The listing builds one solid part. Answer for the finished solid, in the listing's coordinates (mm). A direction names the side the tool comes from. Coordinates: 2 decimals unless noted, no trailing zeros. Write each loop counter-clockwise with the first axis right and the second up, starting at its lowest first coordinate (ties: lowest second). Pieces come first, ordered by that corner, then holes.
Autodesk Inventor part; units mm, degrees
ref_plane "YZ Plane" through (0, 0, 0) normal (1, 0, 0) x (0, 1, 0)
ref_plane "XZ Plane" through (0, 0, 0) normal (0, 1, 0) x (-1, 0, 0)
ref_plane "XY Plane" through (0, 0, 0) normal (0, 0, 1) x (1, 0, 0)
sketch "Sketch1" plane through (0, 0, 0) normal (0, 1, 0) x (-1, 0, 0)
  circle A0 centre (0, 0) radius 10.75
  dimension "d0" = 21.5
extrude "Extrusion1" add sketch "Sketch1" along normal blind 10
sketch "Sketch2" plane through (0, 10, 0) normal (0, 1, 0) x (1, 0, 0)
  circle A0 centre (0, 0) radius 8
  dimension "d3" = 16
extrude "Extrusion2" add sketch "Sketch2" along normal blind 7
sketch "Sketch3" plane through (0, 17, 0) normal (0, 1, 0) x (1, 0, 0)
  circle A0 centre (0, 0) radius 2.5
  dimension "d6" = 5
extrude "Extrusion3" cut sketch "Sketch3" against normal through all
properties part number "Gear drive"
(1) Section C-C, the plane y = 12 is taken. Write down the section's boundary in (x, z), plus the area to 3 significant figures.
(2) Each of these flat-tipped pins is pushed along its axis until it touches: pin 1 (4.5 mm diameter, centred on x = 0, z = 0, fed in from +Y); pin 2 (6 mm diameter, centred on x = 4, y = 11.5, fed in from -Z); pin 3 (3 mm diameter, centred on x = -8.5, z = 6.5, fed in from +Y); pin 4 (2 mm diameter, centred on y = 6, z = 8, fed in from +X). Where does it stop, or does it pass through?
(3) Section A-A, the plane x = 0 is taken. Write down the section's boundary in (y, z), plus the area to 3 significant figures.
(4) Which of the six approach directions +Z, -Z, +X, -X, +Y, -Y give full straight-line access (tool end or side, diameter ignored) to faces 4 (the flat face through (2, 10, 8)), 5 (the flat face through (0, 0, 3))?
(5) Find the intervals of material crossed by probe 1 along Z at (x, y) = (0, 6.5); probe 2 along Z at (x, y) = (0, 12.25), in increasing order.
(6) For a pull along Z with two mould halves and no side action, classify faces 1 (the cylindrical face through (-0.54, 8.62, 2.44)), 2 (the flat face through (-2, 17, 2)), 3 (the cylindrical face through (-1.73, 13.45, -7.81)) as pulls with the +Z half, pulls with the -Z half, needs draft (parallel to the pull), parting line crosses it, or undercut.
(7) Section D-D, the plane z = -3.5 is taken. Write down the section's boundary in (x, y), plus the area to 3 significant figures.
(8) Section B-B, the plane z = 0 is taken. Write down the section's boundary in (x, y).
Solution:
1. outline: circle Ø16 at (0, 0); hole circle Ø5 at (0, 0)
1. area: 181 mm2
2. pin 1: passes through
2. pin 2: stops at z = -10.66
2. pin 3: stops at y = 10
2. pin 4: stops at x = 8.16
3. outline: (0, -10.75) - (10, -10.75) - (10, -8) - (17, -8) - (17, -2.5) - (0, -2.5) - close; (0, 2.5) - (17, 2.5) - (17, 8) - (10, 8) - (10, 10.75) - (0, 10.75) - close
3. area: 242 mm2
4. face 4: +Y
4. face 5: +Z, -Z, +X, -X, -Y
5. probe 1: z = -10.75 to -2.5, 2.5 to 10.75
5. probe 2: z = -8 to -2.5, 2.5 to 8
6. face 1: undercut
6. face 2: needs draft
6. face 3: parting line crosses it
7. outline: (-10.16, 0) - (10.16, 0) - (10.16, 10) - (7.19, 10) - (7.19, 17) - (-7.19, 17) - (-7.19, 10) - (-10.16, 10) - close
7. area: 304 mm2
8. outline: (-10.75, 0) - (-2.5, 0) - (-2.5, 17) - (-8, 17) - (-8, 10) - (-10.75, 10) - close; (2.5, 0) - (10.75, 0) - (10.75, 10) - (8, 10) - (8, 17) - (2.5, 17) - close
